Here's how the part is built. I have some questions about the finished solid (model axes, mm). A direction names the side the tool comes from. Give positions to 0.01 mm unless a question says otherwise; leave off trailing zeros. Loops run counter-clockwise (first coordinate to the right, second up) from the corner with the lowest first, then second, coordinate; pieces in that order, holes last. Notation, with made-up numbers: (22.5, -17.75) -> (59.5, -17.75) arc R8 ccw to (59.5, -8.75) -> close; hole circle Ø2 at (48.5, 6). An arc over 180 degrees is marked (long way). Answer in a Markdown table with one row per item. Add a question column.
Item 1: If I drill on line 1 (Y direction, x = -227.5, z = -127); line 2 (X direction, y = -51, z = -157); line 3 (Y direction, x = -165.5, z = -117.5), over which ranges is the centre line in solid material (lowest first)?
Item 2: For P1, Ø1.5, axis at y = -52.5, z = -27, coming from the -X side; P2, Ø8, axis at x = -171.5, z = -10.5, coming from the -Y side, each with a flat end and sliding along its axis, tell me the tip position at first contact or that it passes through.
Item 3: If we section it at A-A (x = -196): Write out the boundary of the cut face in (y, z), then the cut area to 3 significant figures.
Item 4: If we section it at C-C (z = -68): Write out the boundary of the cut face in (x, y).
Item 5: If we section it at D-D (y = -23.5): Write out the boundary of the cut face in (x, z).
Item 6: If we section it at B-B (z = 157.8): Write out the boundary of the cut face in (x, y).
Item 7: Which directions (+Z, -Z, +X, -X, +Y, -Y) give clear straight access to the entire face, cutting with the end or side of a thin tool? Please do faces 1 (the face through (-218, -67.631, -2)), 2 (the face through (-153.924, -29, -2)).
```python
from build123d import *

# Parameters (mm, degrees)
CROQUIS2_W                                           = 95.38
CROQUIS2_H                                           = 352.6
BRIDA_BASE1_DEPTH                                    = 1.5
BRIDA_DE_ARISTA1_STRIP_W                             = 16
BRIDA_DE_ARISTA1_STRIP_H                             = 1.5
BRIDA_DE_ARISTA1_STRIP_CUT_DEPTH                     = 352.6
BRIDA_DE_ARISTA1_DEPTH                               = 352.6
BRIDA_START                                          = -176.3
BRIDA_DE_ARISTA2_DEPTH                               = 352.6
BRIDA_DE_ARISTA2_2_DEPTH                             = 352.6
BRIDA_DE_ARISTA3_DEPTH                               = 352.6
BRIDA_DE_ARISTA3_2_DEPTH                             = 352.6
CROQUIS22_R                                          = 2.25
CORTAR_EXTRUIR4_DEPTH                                = 312.548097
AVELLANADO_PARA_TORNILLO_CON_CABEZA_PLAN_D           = 5.5
AVELLANADO_PARA_TORNILLO_CON_CABEZA_PLAN_CSINK_D     = 10.4
AVELLANADO_PARA_TORNILLO_CON_CABEZA_PLAN_CSINK_ANGLE = 90
AVELLANADO_PARA_TORNILLO_CON_CABEZA_2_D              = 5.5
AVELLANADO_PARA_TORNILLO_CON_CABEZA_2_CSINK_D        = 10.4
AVELLANADO_PARA_TORNILLO_CON_CABEZA_2_CSINK_ANGLE    = 90


# Read off the part's stored shape, not the designer's step: Brida de arista2, Brida de arista3
# Sheet-metal steps are written as plain solids
with BuildPart() as part:
    # Croquis2 → Brida base1 (new body)
    with BuildSketch(Plane(origin=(0, 0, 0), x_dir=(1, 0, 0), z_dir=(0, 1, 0))):
        with Locations((-200.113558854, 0)):
            Rectangle(CROQUIS2_W, CROQUIS2_H)
    extrude(amount=-BRIDA_BASE1_DEPTH)

    # Brida de arista1 strip (across the edge) → Brida de arista1 strip cut (cut)
    with BuildSketch(Plane(origin=(-152.423558854, -1.5, -176.3), x_dir=(-1, 0, 0), z_dir=(0, 0, 1))):
        with Locations((-1.5, -0.75)):
            Rectangle(BRIDA_DE_ARISTA1_STRIP_W, BRIDA_DE_ARISTA1_STRIP_H)
    extrude(amount=BRIDA_DE_ARISTA1_STRIP_CUT_DEPTH, mode=Mode.SUBTRACT)

    # Brida de arista1 section (across the edge) → Brida de arista1 (add)
    with BuildSketch(Plane(origin=(-152.423558854, -1.5, -176.3), x_dir=(-1, 0, 0), z_dir=(0, 0, 1))):
        with BuildLine():
            Line((0, 5), (0, 54.19))
            Line((0, 54.19), (1.5, 54.19))
            Line((1.5, 54.19), (1.5, 5))
            ThreePointArc((1.5, 5), (2.964466094, 1.464466094), (6.5, 0))
            Line((6.5, 0), (6.5, -1.5))
            ThreePointArc((6.5, -1.5), (1.903805922, 0.403805922), (0, 5))
        make_face()
    extrude(amount=BRIDA_DE_ARISTA1_DEPTH)

    # Brida de arista2 outline → Brida de arista2 (cut)
    with BuildSketch(Plane.XY.offset(BRIDA_START)):
        with BuildLine():
            ThreePointArc((-152.423558854, -50.59269565), (-152.810049223, -52.800635867), (-153.923558854, -54.746007582))
            Line((-153.923558854, -54.746007582), (-153.923558854, -55.69))
            Line((-153.923558854, -55.69), (-152.423558854, -55.69))
            Line((-152.423558854, -55.69), (-152.423558854, -50.59269565))
        make_face()
    extrude(amount=BRIDA_DE_ARISTA2_DEPTH, mode=Mode.SUBTRACT)

    # Brida de arista2 2 outline → Brida de arista2 2 (add)
    with BuildSketch(Plane.XY.offset(BRIDA_START)):
        with BuildLine():
            Line((-190.603270036, -69.040323072), (-156.700427922, -56.700697685))
            ThreePointArc((-156.700427922, -56.700697685), (-155.182087424, -55.90789946), (-153.923558854, -54.746007582))
            Line((-153.923558854, -54.746007582), (-153.923558854, -50.59269565))
            ThreePointArc((-153.923558854, -50.59269565), (-154.827798632, -53.460577832), (-157.213458137, -55.291158754))
            Line((-157.213458137, -55.291158754), (-191.116300251, -67.630784141))
            Line((-191.116300251, -67.630784141), (-190.603270036, -69.040323072))
        make_face()
    extrude(amount=BRIDA_DE_ARISTA2_2_DEPTH)

    # Brida de arista3 outline → Brida de arista3 (cut)
    with BuildSketch(Plane.XY.offset(BRIDA_START)):
        with BuildLine():
            Line((-187.876719026, -67.630784141), (-191.116300251, -67.630784141))
            Line((-191.116300251, -67.630784141), (-190.603270036, -69.040323072))
            Line((-190.603270036, -69.040323072), (-185.653588094, -67.238786176))
            ThreePointArc((-185.653588094, -67.238786176), (-186.748005871, -67.532034535), (-187.876719026, -67.630784141))
        make_face()
    extrude(amount=BRIDA_DE_ARISTA3_DEPTH, mode=Mode.SUBTRACT)

    # Brida de arista3 2 outline → Brida de arista3 2 (add)
    with BuildSketch(Plane.XY.offset(BRIDA_START)):
        with BuildLine():
            Line((-247.803558854, -66.130784141), (-247.803558854, -67.630784141))
            Line((-247.803558854, -67.630784141), (-191.116300251, -67.630784141))
            Line((-191.116300251, -67.630784141), (-186.166618309, -65.829247245))
            ThreePointArc((-186.166618309, -65.829247245), (-187.008478137, -66.054822906), (-187.876719026, -66.130784141))
            Line((-187.876719026, -66.130784141), (-247.803558854, -66.130784141))
        make_face()
    extrude(amount=BRIDA_DE_ARISTA3_2_DEPTH)

    # Croquis22 → Cortar-Extruir4 (cut, through all)
    with BuildSketch(Plane.XZ):
        with Locations(Location((-239.303558854, 157.8, 0), (0, 0, 180))):
            Circle(CROQUIS22_R)
        with Locations(Location((-239.303558854, 51.733333333, 0), (0, 0, 180))):
            Circle(CROQUIS22_R)
        with Locations(Location((-239.303558854, -54.333333333, 0), (0, 0, 180))):
            Circle(CROQUIS22_R)
        with Locations(Location((-239.303558854, -160.4, 0), (0, 0, 180))):
            Circle(CROQUIS22_R)
    extrude(amount=CORTAR_EXTRUIR4_DEPTH, mode=Mode.SUBTRACT)

    # Avellanado para tornillo con cabeza plan (through all)
    with Locations(Plane(origin=(0, 0, 0), x_dir=(1, 0, 0), z_dir=(0, 1, 0))):
        with Locations((-239.303558854, 160.4), (-239.303558854, 54.333333333), (-239.303558854, -51.733333333), (-239.303558854, -157.8)):
            CounterSinkHole(AVELLANADO_PARA_TORNILLO_CON_CABEZA_PLAN_D / 2, AVELLANADO_PARA_TORNILLO_CON_CABEZA_PLAN_CSINK_D / 2, counter_sink_angle=AVELLANADO_PARA_TORNILLO_CON_CABEZA_PLAN_CSINK_ANGLE)

    # Avellanado para tornillo con cabeza  2 (through all)
    with Locations(Plane(origin=(0, -67.630784141, 0), x_dir=(-1, 0, 0), z_dir=(0, -1, 0))):
        with Locations((239.303558854, 160.4), (239.303558854, 54.333333333), (239.303558854, -51.733333333), (239.303558854, -157.8)):
            CounterSinkHole(AVELLANADO_PARA_TORNILLO_CON_CABEZA_2_D / 2, AVELLANADO_PARA_TORNILLO_CON_CABEZA_2_CSINK_D / 2, counter_sink_angle=AVELLANADO_PARA_TORNILLO_CON_CABEZA_2_CSINK_ANGLE)


solid = part.part
```
Recorded:
| question | item | result |
|---|---|---|
| 1 | line 1 | y = -67.63 to -66.13, -1.5 to 0 |
| 1 | line 2 | x = -153.94 to -152.44 |
| 1 | line 3 | y = -59.9 to -58.31, -1.5 to 0 |
| 2 | P1 | stops at x = -154.69 |
| 2 | P2 | stops at y = -63.54 |
| 3 | outline | (-67.63, -176.3) -> (-66.13, -176.3) -> (-66.13, 176.3) -> (-67.63, 176.3) -> close; (-1.5, -176.3) -> (0, -176.3) -> (0, 176.3) -> (-1.5, 176.3) -> close |
| 3 | area | 1,060 mm^2 |
| 4 | outline | (-247.8, -67.63) -> (-187.88, -67.63) arc R6.5 ccw to (-185.65, -67.24) -> (-156.7, -56.7) arc R6.5 ccw to (-152.42, -50.59) -> (-152.42, -6.5) arc R6.5 ccw to (-158.92, 0) -> (-247.8, 0) -> (-247.8, -1.5) -> (-158.92, -1.5) arc R5 cw to (-153.92, -6.5) -> (-153.92, -50.59) arc R5 cw to (-157.21, -55.29) -> (-186.17, -65.83) arc R5 cw to (-187.88, -66.13) -> (-247.8, -66.13) -> close |
| 5 | outline | (-153.92, -176.3) -> (-152.42, -176.3) -> (-152.42, 176.3) -> (-153.92, 176.3) -> close |
| 6 | outline | (-247.8, -67.63) -> (-244.5, -67.63) -> (-243, -66.13) -> (-247.8, -66.13) -> close; (-247.8, -1.5) -> (-243, -1.5) -> (-244.5, 0) -> (-247.8, 0) -> close; (-235.6, -66.13) -> (-234.1, -67.63) -> (-187.88, -67.63) arc R6.5 ccw to (-185.65, -67.24) -> (-156.7, -56.7) arc R6.5 ccw to (-152.42, -50.59) -> (-152.42, -6.5) arc R6.5 ccw to (-158.92, 0) -> (-234.1, 0) -> (-235.6, -1.5) -> (-158.92, -1.5) arc R5 cw to (-153.92, -6.5) -> (-153.92, -50.59) arc R5 cw to (-157.21, -55.29) -> (-186.17, -65.83) arc R5 cw to (-187.88, -66.13) -> close |
| 7 | face 1 | +Z, -Z, +X, -X, -Y |
| 7 | face 2 | +Z, -Z, -X |
